Input: dimensioned drawing with shaded views. Units: mm. Origin: part minimum x, y, z. A direction names the side the tool comes from. Round coordinates to 2 decimals unless told otherwise and drop trailing zeros. Write each loop counter-clockwise with the first axis right and the second up, starting at its lowest first coordinate (ties: lowest second). Pieces come first, ordered by that corner, then holes. Notation, with made-up numbers: (24.5, -25) -> (75.5, -25) arc R36 ccw to (75.5, 13) -> close; hole circle Ø7 at (80.5, 20.25). An arc over 180 degrees is marked (long way). Use one line per item in the form item = value. Start each with the question number.
1. Pin query (flat end, axial travel): pin 1 Ø16.5 at (x, z) = (105, 66) entering from +Y; pin 2 Ø18.5 at (y, z) = (29.5, 45.5) entering from -X; pin 3 Ø5.5 at (x, z) = (8, 31) entering from -Y. Return the tip coordinate at first contact, or that it passes through.
2. Cut plane A-A, the plane x = 102. Return the cut outline in (y, z) (3 decimals), plus the area to 3 significant figures.
3. Cut plane B-B, the plane z = 66. Return the cut outline in (x, y) (3 decimals), plus the area to 3 significant figures.
4. Cut plane C-C, the plane z = 84. Return the cut outline in (x, y).
5. Reachability of the marked faces 1, 2 and 3 from +Z, -Z, +X, -X, +Y, -Y: full face, straight path, thin tool, end or side. Return the list, or none.
6. Line query: L1, parallel to Z at x = 8, y = 7.25 (3 decimals); L2, parallel to X at y = 9, z = 31 (3 decimals); L3, parallel to X at y = 37, z = 67. Output: solid intervals per line, ascending.
7. Cut plane D-D, the plane y = 34.5. Return the cut outline in (x, z).
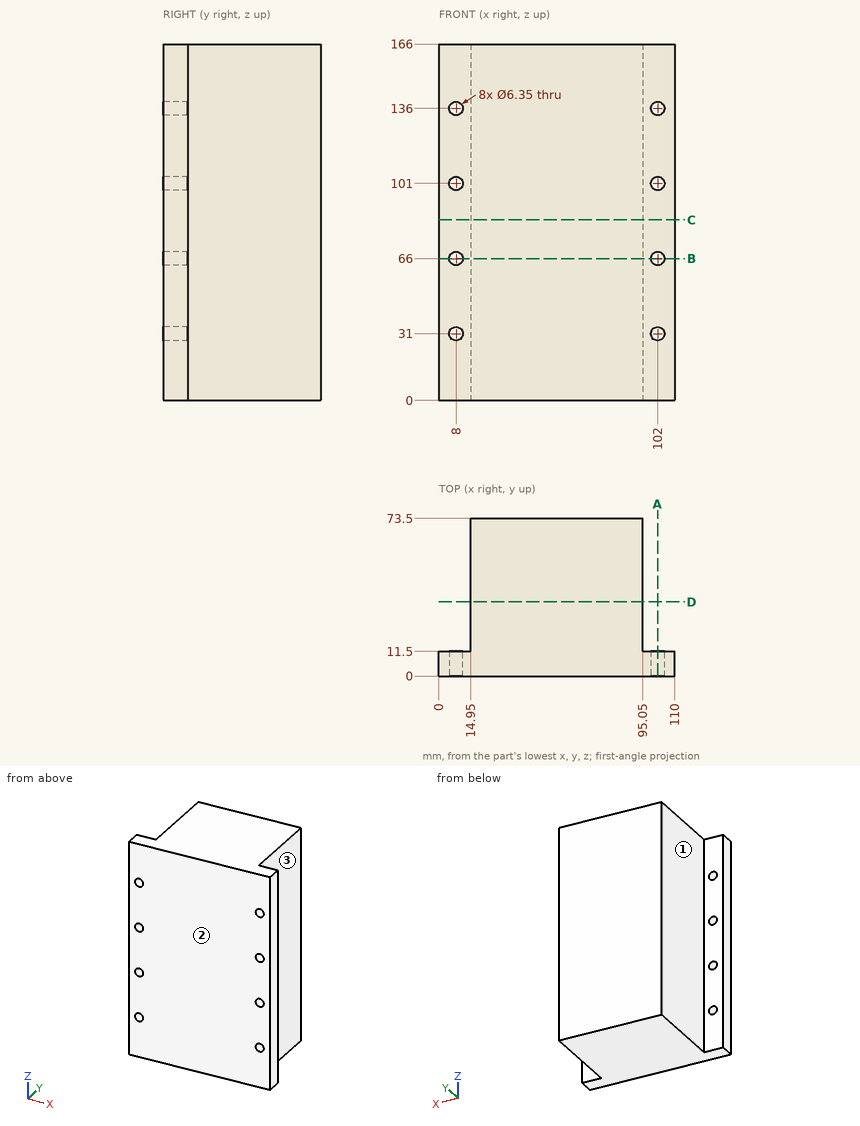
Outcome:
q1.pin_1 = 11.5
q1.pin_2 = 14.95
q1.pin_3 = through
q2.outline = (0, 0) -> (11.5, 0) -> (11.5, 27.825) -> (0, 27.825) -> close; (0, 34.175) -> (11.5, 34.175) -> (11.5, 62.825) -> (0, 62.825) -> close; (0, 69.175) -> (11.5, 69.175) -> (11.5, 97.825) -> (0, 97.825) -> close; (0, 104.175) -> (11.5, 104.175) -> (11.5, 132.825) -> (0, 132.825) -> close; (0, 139.175) -> (11.5, 139.175) -> (11.5, 166) -> (0, 166) -> close
q2.area = 1,620 mm^2
q3.outline = (0, 0) -> (4.825, 0) -> (4.825, 11.5) -> (0, 11.5) -> close; (11.175, 0) -> (98.825, 0) -> (98.825, 11.5) -> (95.05, 11.5) -> (95.05, 73.5) -> (14.95, 73.5) -> (14.95, 11.5) -> (11.175, 11.5) -> close; (105.175, 0) -> (110, 0) -> (110, 11.5) -> (105.175, 11.5) -> close
q3.area = 6,090 mm^2
q4.outline = (0, 0) -> (110, 0) -> (110, 11.5) -> (95.05, 11.5) -> (95.05, 73.5) -> (14.95, 73.5) -> (14.95, 11.5) -> (0, 11.5) -> close
q5.face_1 = +Z, -Z, -X, +Y
q5.face_2 = +Z, -Z, +X, -X, -Y
q5.face_3 = +Z, -Z, +X, +Y
q6.L1 = 0 to 27.825, 34.175 to 62.825, 69.175 to 97.825, 104.175 to 132.825, 139.175 to 166
q6.L2 = 0 to 4.825, 11.175 to 98.825, 105.175 to 110
q6.L3 = 14.95 to 95.05
q7.outline = (14.95, 0) -> (95.05, 0) -> (95.05, 166) -> (14.95, 166) -> close
